```python
from build123d import *

# Parameters (mm, degrees)
SKETCH2_W          = 5.424806346
SKETCH2_H          = 1.2
CUT_EXTRUDE1_DEPTH = 2


with BuildPart() as part:
    # Sketch1 → Revolve1 (revolve)
    with BuildSketch(Plane(origin=(0, 0, 0), x_dir=(0, 0, -1), z_dir=(1, 0, 0)), mode=Mode.PRIVATE) as revolve1_sk:
        Polygon((0, 0), (0, 2), (0.5, 2.5), (17, 2.5), (17, 0), align=None)
    revolve(revolve1_sk.sketch.rotate(Axis((0, 0, 0), (0, 0, -1)), 90), axis=Axis((0, 0, 0), (0, 0, -1)))

    # Sketch2 → Cut-Extrude1 (cut)
    with BuildSketch(Plane(origin=(0, 0, -17), x_dir=(-1, 0, 0), z_dir=(0, 0, -1))):
        Rectangle(SKETCH2_W, SKETCH2_H)
    extrude(amount=-CUT_EXTRUDE1_DEPTH, mode=Mode.SUBTRACT)


solid = part.part
```
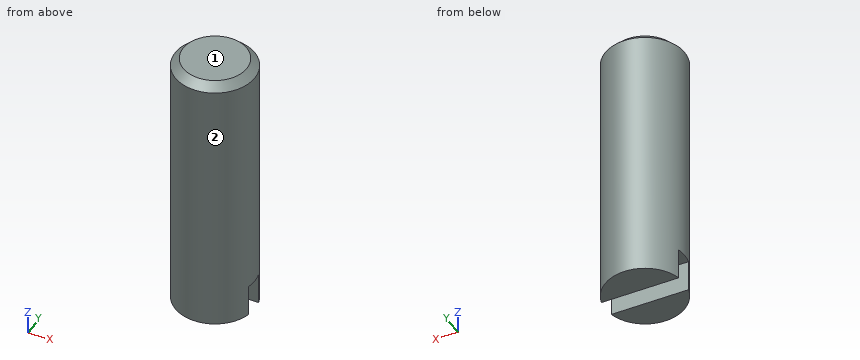
Here's how the part is built. I have some questions about the finished solid (model axes, mm). Face numbers are marked on the shaded views. Give positions to 0.01 mm unless a question says otherwise; leave off trailing zeros. Order: outer loops, then holes, each group sorted by start corner. A loop starts at its lowest first (then second) coordinate and runs counter-clockwise, first axis right, second up. Notation, with made-up numbers: (73, -38) -> (101, -38) arc R25 ccw to (101, -26) -> close; hole circle Ø11 at (-17.75, -25.75). An arc over 180 degrees is marked (long way). Use CSV: the item, a comma, the result in double quotes. Start each with the question number.
Item 1: If I drill on probe 1 along Y at (x, z) = (-0.45, -15.5); probe 2 along Z at (x, y) = (0.5, 0.2); probe 3 along Y at (x, z) = (1.4, -15.25), over which ranges is the centre line in solid material (lowest first)? Write a range as [from, to].
Item 2: Suppose I cut it at A-A (x = 0). List the corners of the cut face in (y, z) for me, and give its area (4 significant figures).
Item 3: Suppose I cut it at C-C (z = -4.25). List the corners of the cut face in (x, y) for me.
Item 4: Thinking about a two-plate mould opening in Y: for the marked faces 1 and 2, which applies, pulls with the +Y half, pulls with the -Y half, needs draft (parallel to the pull), parting line crosses it, or undercut?
Item 5: I'm going to push flat-ended pins straight in: P1, Ø1, axis at x = -2, z = -2, coming from the -Y side; P2, Ø1, axis at y = 1.5, z = -3, coming from the -X side. Where does each tip first touch, or does it pass through?
Item 6: Suppose I cut it at B-B (y = 0). List the corners of the cut face in (x, z) for me.
Answer block:
1,probe 1,"y = [-2.46, -0.6], [0.6, 2.46]"
1,probe 2,"z = [-15, 0]"
1,probe 3,"y = [-2.07, -0.6], [0.6, 2.07]"
2,outline,"(-2.5, -17) -> (-0.6, -17) -> (-0.6, -15) -> (0.6, -15) -> (0.6, -17) -> (2.5, -17) -> (2.5, -0.5) -> (2, 0) -> (-2, 0) -> (-2.5, -0.5) -> close"
2,area,"82.35 mm^2"
3,outline,"circle Ø5 at (0, 0)"
4,face 1,"needs draft"
4,face 2,"parting line crosses it"
5,P1,"stops at y = -2"
5,P2,"stops at x = -2.29"
6,outline,"(-2.5, -15) -> (2.5, -15) -> (2.5, -0.5) -> (2, 0) -> (-2, 0) -> (-2.5, -0.5) -> close"
